Verification items for the finished model (mm, model axes). Face numbers are marked on the shaded views. A direction names the side the tool comes from. Round coordinates to 2 decimals unless told otherwise and drop trailing zeros. Write each loop counter-clockwise with the first axis right and the second up, starting at its lowest first coordinate (ties: lowest second). Pieces come first, ordered by that corner, then holes. Notation, with made-up numbers: M 59,-7.5 L 100,-7.5 A16 ccw 100,9.5 Z; hole C 3,17.5 d3. An arc over 180 degrees is marked long. Write each question's results on one line, items separated by ' | '.
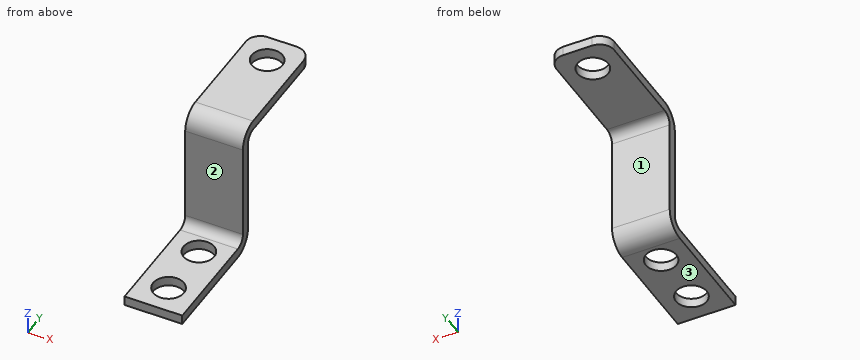
Autodesk Inventor part; units mm, degrees
ref_plane "YZ Plane" through (0, 0, 0) normal (1, 0, 0) x (0, 1, 0)
ref_plane "XZ Plane" through (0, 0, 0) normal (0, 1, 0) x (-1, 0, 0)
ref_plane "XY Plane" through (0, 0, 0) normal (0, 0, 1) x (1, 0, 0)
sketch "Sketch5" plane through (-3, 6, 14) normal (0, -1, 0) x (1, 0, 0)
  circle A0 centre (3, -8) radius 1.6
  circle A1 centre (3, -3) radius 1.6
  line L0 (6, 0) -> (0, 0)
  point P0 (3, -14)
  point P1 (3, 0)
  dimension "d33" = 3.2
  dimension "d34" = 3.2
  dimension "d35" = 5
  dimension "d36" = 3
sketch "Sketch1" plane through (0, 0, 0) normal (0, 0, 1) x (1, 0, 0)
  line L0 (-3, 6) -> (3, 6)
  line L1 (3, 6) -> (3, -6)
  line L2 (3, -6) -> (-3, -6)
  line L3 (-3, -6) -> (-3, 6)
  line L4 (-3, 6) -> (3, -6) construction
  line L5 (3, 6) -> (-3, -6) construction
  circle A0 centre (0, 3) radius 1.6
  circle A1 centre (0, -3) radius 1.6
  point P0 (0, 0)
  dimension "d0" = 12
  dimension "d1" = 6
  dimension "d2" = 3.2
  dimension "d3" = 3.2
  dimension "d4" = 6
  dimension "d5" = 3
extrude "Plate1" add sketch "Sketch1" along normal blind 1
sketch "Sketch2" plane through (-3, 6, 1) normal (0, 1, 0) x (-1, 0, 0)
  line L0 (-6, 0) -> (0, 0)
  line L1 (0, 0) -> (0, 13)
  line L2 (0, 13) -> (-6, 13)
  line L3 (-6, 13) -> (-6, 0)
edge flange "Flange1" height 14 angle 90 thickness 1 bend radius 1 thickness toward (0, 1, 0) relief tear relief width 1 relief depth 0.5 edges at (0, 6, 1) wall of the first edge with corners at (3, 6, 1) (-3, 6, 1) (-3, 6, 14) (3, 6, 14)
bend "Bend1"
corner "Corner1"
sketch "Sketch6" plane through (3, 6, 13) normal (0, 0, 1) x (1, 0, 0)
  line L0 (-6, 0) -> (0, 0)
  line L1 (0, 0) -> (0, 13.5)
  line L2 (0, 13.5) -> (-6, 13.5)
  line L3 (-6, 13.5) -> (-6, 0)
edge flange "Flange3" height 13.5 angle 90 thickness 1 bend radius 1 thickness toward (0, 0, 1) relief tear relief width 1 relief depth 0.5 edges at (0, 7, 14) wall of the first edge with corners at (-3, 6, 13) (3, 6, 13) (3, 19.5, 13) (-3, 19.5, 13)
bend "Bend3"
corner "Corner3"
fillet "Corner Round1" radius 1.5 2 edges at (3, 19.5, 13.5) (-3, 19.5, 13.5)
sketch "Sketch7" plane through (-3, 8, 14) normal (0, 0, 1) x (1, 0, 0)
  circle A0 centre (3, 8.5) radius 1.6
  line L0 (0, 0) -> (6, 0)
  line L1 (1.5, 11.5) -> (4.5, 11.5)
  point P0 (3, -8)
  point P1 (3, 0)
  dimension "d50" = 3.2
  dimension "d51" = 3
extrude "Cut3" cut sketch "Sketch7" against normal blind 1
equation "\"d52\" = 厚度"
equation "\"d6\" = 厚度"
equation "\"d7\" = 折彎離隙寬度"
equation "\"d8\" = 折彎離隙深度"
equation "\"d9\" = 最小剩餘"
equation "\"d10\" = 轉移半徑"
equation "\"d13\" = 折彎半徑"
equation "\"d14\" = 轉角離隙大小"
equation "\"d15\" = 間隙大小"
equation "\"d16\" = Jacobi半徑大小"
equation "\"d39\" = 折彎離隙寬度"
equation "\"d40\" = 折彎離隙深度"
equation "\"d41\" = 最小剩餘"
equation "\"d42\" = 轉移半徑"
equation "\"d45\" = 折彎半徑"
equation "\"d46\" = 轉角離隙大小"
equation "\"d47\" = 間隙大小"
equation "\"d48\" = Jacobi半徑大小"
equation "\"折彎半徑\" = 厚度"
equation "\"折彎離隙寬度\" = 厚度"
equation "\"折彎離隙深度\" = 0.5 * 厚度"
equation "\"轉角離隙大小\" = 4 * 厚度"
equation "\"最小剩餘\" = 2 * 厚度"
equation "\"轉移半徑\" = 折彎半徑"
equation "\"Jacobi半徑大小\" = 折彎半徑"
equation "\"間隙大小\" = 厚度"
properties part number "connector_Zshape"
1) Material ranges on line 1 (Y direction, x = 0, z = 0.85); line 2 (Y direction, x = 0, z = 0.3); line 3 (Z direction, x = -1.8, y = 0.75), recorded low to high. Write a range as [from, to].
Calculated:
line 1: y = [-6, -4.6], [-1.4, 1.4], [4.6, 6.64] | line 2: y = [-6, -4.6], [-1.4, 1.4], [4.6, 6.05] | line 3: z = [0, 1]
2) Sectioned sample at B-B, the plane x = 0. Record the cut outline in (y, z), and give its area (3 significant figures).
Calculated:
outline: M -6,0 L -4.6,0 L -4.6,1 L -6,1 Z; M -1.4,0 L 1.4,0 L 1.4,1 L -1.4,1 Z; M 4.6,0 L 5,0 A2 ccw 7,2 L 7,12 A1 cw 8,13 L 14.9,13 L 14.9,14 L 8,14 A2 ccw 6,12 L 6,2 A1 cw 5,1 L 4.6,1 Z; M 18.1,13 L 19.5,13 L 19.5,14 L 18.1,14 Z | area: 27.6 mm²
3) Access from +Z, -Z, +X, -X, +Y, -Y to the whole of each face (thin tool, end or side, straight path). Record for the marked faces 1, 2 and 3.
Calculated:
face 1: -Z, +X, -X, +Y | face 2: +Z, +X, -X, -Y | face 3: -Z, +X, -X, +Y, -Y
4) Sectioned sample at A-A, the plane y = -3. Record the cut outline in (x, z), and give its area (3 significant figures).
Calculated:
outline: M -3,0 L -1.6,0 L -1.6,1 L -3,1 Z; M 1.6,0 L 3,0 L 3,1 L 1.6,1 Z | area: 2.80 mm²
5) Sectioned sample at C-C, the plane z = 7.75. Record the cut outline in (x, y).
Calculated:
outline: M -3,6 L 3,6 L 3,7 L -3,7 Z
6) Sectioned sample at D-D, the plane y = 8.5. Record the cut outline in (x, z).
Calculated:
outline: M -3,13 L 3,13 L 3,14 L -3,14 Z
7) Depth check by flat-ended pin: P1, Ø1.8, axis at x = 0, z = 7, coming from the -Y side; P2, Ø1.8, axis at x = -1, y = -3, coming from the +Z side; P3, Ø1.8, axis at x = 0.5, y = 11, coming from the -Z side; P4, Ø3, axis at x = 2, y = 2, coming from the -Z side. Enter the tip coordinate at first touch or a pass-through.
Calculated:
P1: stops at y = 6 | P2: stops at z = 1 | P3: stops at z = 13 | P4: stops at z = 0
